Solid Edge part; units mm, degrees
sketch "Sketch1" plane through (0, 0, 0) normal (0, -1, 0) x (1, 0, 0)
  line L0 (0, 72) -> (0, 0)
  line L1 (0, 0) -> (145, 0)
  line L2 (145, 0) -> (145, 72)
  line L3 (145, 72) -> (0, 72)
extrude "Protrusion1" add sketch "Sketch1" against normal blind 25
sketch "Sketch2" plane through (0, 0, 0) normal (0, -1, 0) x (1, 0, 0)
  line L0 (36, 0) -> (36, 72)
  line L1 (36, 72) -> (0, 72)
  line L2 (0, 72) -> (0, 0)
  line L3 (0, 0) -> (36, 0)
extrude "ExtrudedProtrusion_2" add sketch "Sketch2" against normal blind 90
sketch "Sketch3" plane through (90.5, 25, 36) normal (0, 1, 0) x (1, 0, 0)
  line L0 (54.5, 12) -> (4.5, 12)
  line L1 (54.5, -12) -> (54.5, 12)
  line L2 (4.5, -12) -> (54.5, -12)
  arc A0 (4.5, -12) -> (4.5, 12) centre (4.5, 0) cw
extrude "ExtrudedCutout_1" cut sketch "Sketch3" against normal blind 25 and the other way blind 1
sketch "Sketch4" plane through (0, 45, 36) normal (-1, 0, 0) x (0, 1, 0)
  circle A0 centre (4, 0) radius 12
  circle A1 centre (4, 0) radius 30
extrude "ExtrudedCutout_5" cut sketch "Sketch4" against normal blind 12 and the other way blind 1
sketch "Sketch5" plane through (0, 49, 36) normal (-1, 0, 0) x (0, 1, 0)
  circle A0 centre (0, 0) radius 12
extrude "ExtrudedCutout_6" cut sketch "Sketch5" against normal blind 36 and the other way blind 1
sketch "Sketch6" plane through (0, 45, 36) normal (-1, 0, 0) x (0, 1, 0)
  line L0 (4, 36) -> (22, 36)
  line L1 (22, 36) -> (22, 24)
  arc A0 (22, 24) -> (-14, 24) centre (4, 0) ccw
  line L2 (-14, 36) -> (-14, 24)
  line L3 (4, 36) -> (-14, 36)
  line L4 (4, -36) -> (22, -36)
  line L5 (22, -36) -> (22, -24)
  arc A1 (22, -24) -> (-14, -24) centre (4, 0) cw
  line L6 (-14, -36) -> (-14, -24)
  line L7 (4, -36) -> (-14, -36)
extrude "ExtrudedCutout_7" cut sketch "Sketch6" against normal blind 12 and the other way blind 1
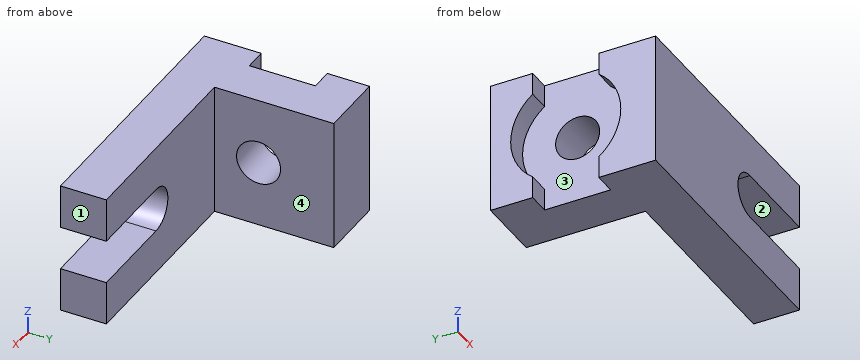
Source: CAD feature listing. Evaluate the final solid. Frame: model axes, mm. Face numbers are marked on the shaded views. A direction names the side the tool comes from. Coordinates: 2 decimals unless noted, no trailing zeros. Order: outer loops, then holes, each group sorted by start corner. A loop starts at its lowest first (then second) coordinate and runs counter-clockwise, first axis right, second up. Notation, with made-up numbers: M 40,-40 L 98,-40 A15 ccw 98,-20 Z; hole C 9,78 d8. An arc over 180 degrees is marked long. Write each question's results on one line, items separated by ' | '. Start each with the question number.
1. Pin query (flat end, axial travel): pin 1 (8 mm diameter, centred on y = 38.5, z = 10.5, fed in from -X); pin 2 (1.5 mm diameter, centred on y = 26, z = 63, fed in from +X). Return the tip coordinate at first contact, or that it passes through.
2. Section D-D, the plane z = 62.5. Return the cut outline in (x, y).
3. Reachability of the marked faces 1, 2, 3 and 4 from +Z, -Z, +X, -X, +Y, -Y: full face, straight path, thin tool, end or side. Return the list, or none.
4. Section B-B, the plane y = 49. Return the cut outline in (x, z).
5. Section C-C, the plane x = 19. Return the cut outline in (y, z).
6. Section A-A, the plane z = 36. Return the cut outline in (x, y), then the cut area to 3 significant figures.
7. Material intervals for L1, parallel to Z at x = 22, y = 49; L2, parallel to Y at x = 29, z = 36; L3, parallel to X at y = 79.5, z = 41, sorted ascending.
Solution:
1) pin 1: x = 12 | pin 2: x = 36
2) outline: M 0,0 L 145,0 L 145,25 L 36,25 L 36,90 L 0,90 L 0,67 L 12,67 L 12,31 L 0,31 Z
3) face 1: +Z, -Z, +X, +Y, -Y | face 2: +X, +Y, -Y | face 3: -X | face 4: +Z, -Z, +X, +Y
4) outline: M 12,0 L 36,0 L 36,24 L 12,24 Z; M 12,48 L 36,48 L 36,72 L 12,72 Z
5) outline: M 0,0 L 90,0 L 90,72 L 0,72 Z; hole C 49,36 d24
6) outline: M 0,0 L 83,0 L 83,25 L 36,25 L 36,37 L 12,37 L 12,19 L 0,19 Z; M 0,79 L 12,79 L 12,61 L 36,61 L 36,90 L 0,90 Z | area: 3,120 mm²
7) L1: 0 to 24, 48 to 72 | L2: 0 to 37, 61 to 90 | L3: 0 to 36
